from build123d import *

# Parameters (mm, degrees)
BOSS_EXTRUDE1_DEPTH = 17.5
FILLET1_R           = 2
SKETCH3_W           = 5
SKETCH3_H           = 7.5
CUT_EXTRUDE1_DEPTH  = 66


with BuildPart() as part:
    # Sketch2 → Boss-Extrude1 (new body, symmetric)
    with BuildSketch(Plane(origin=(0, 0, 0), x_dir=(1, 0, 0), z_dir=(0, 1, 0))):
        with BuildLine():
            Line((5.25, 14.75), (5.25, -14.75))
            ThreePointArc((5.25, -14.75), (0, -20), (5.25, -25.25))
            Line((5.25, -25.25), (5.25, -32.5))
            Line((5.25, -32.5), (-14.75, -32.5))
            Line((-14.75, -32.5), (-14.75, 32.5))
            Line((-14.75, 32.5), (5.25, 32.5))
            Line((5.25, 32.5), (5.25, 25.25))
            ThreePointArc((5.25, 25.25), (0, 20), (5.25, 14.75))
        make_face()
    extrude(amount=BOSS_EXTRUDE1_DEPTH, both=True)

    # Fillet1
    fillet1_edges = [part.edges().sort_by_distance(p)[0] for p in [
        (-14.75, -17.5, 0),
        (-4.75, -17.5, -32.5),
        (5.25, -17.5, -28.875),
        (0, -17.5, -20),
        (-4.75, 17.5, -32.5),
        (5.25, 0, 32.5),
        (-14.75, 0, 32.5),
        (-14.75, 0, -32.5),
        (5.25, 0, -32.5),
        (-14.75, 17.5, 0),
        (-4.75, 17.5, 32.5),
        (5.25, 17.5, 28.875),
        (0, 17.5, 20),
        (5.25, 17.5, 0),
        (0, 17.5, -20),
        (5.25, -17.5, 0),
        (5.25, 17.5, -28.875),
        (0, -17.5, 20),
        (5.25, -17.5, 28.875),
        (-4.75, -17.5, 32.5),
    ]]
    fillet(fillet1_edges, radius=FILLET1_R)

    # Sketch3 → Cut-Extrude1 (cut, through all)
    with BuildSketch(Plane.XY.offset(32.5)):
        with Locations((-12.25, 0)):
            Rectangle(SKETCH3_W, SKETCH3_H)
    extrude(amount=-CUT_EXTRUDE1_DEPTH, mode=Mode.SUBTRACT)


solid = part.part
Geometry: final body of the model. Coordinates: model frame, mm. A direction names the side the tool comes from. Give positions to 0.01 mm unless a question says otherwise; leave off trailing zeros. Write each loop counter-clockwise with the first axis right and the second up, starting at its lowest first coordinate (ties: lowest second). Pieces come first, ordered by that corner, then holes. Notation, with made-up numbers: (-30, 36) - (-2, 36) arc R20 ccw to (-2, 48) - close; hole circle Ø3 at (-10, 8.25). An arc over 180 degrees is marked (long way). Return JSON: item names as keys, results as strings. Group by question number.
1) Set-up query: faces 1 (the flat face through (-14.75, 10, 0)), 2 (the flat face through (-9.75, 0, 0)). Return all of +Z, -Z, +X, -X, +Y, -Y with unobstructed straight access to the full face (end or side cutting, diameter ignored); none if empty.
2) Section A-A on x = -11.5. Return the cut outline in (y, z).
3) Section D-D on y = -1. Return the cut outline in (x, z), plus the area to 3 significant figures.
4) First-contact query: P1, Ø4, axis at y = 1.5, z = -7.5, coming from the -X side. Flat tip, straight axial feed; report the tip coordinate or a pass-through.
5) Line query: line 1 (Z direction, x = 0.75, y = -12); line 2 (Z direction, x = 2.75, y = 8); line 3 (Y direction, x = -11.5, z = 18). Output: solid intervals per line, ascending.
6) Section B-B on z = -2. Return the cut outline in (x, y).
7) Section C-C on y = -6. Return the cut outline in (x, z).
Filled in:
{
 "1": {"face 1": "+Z, -Z, -X, +Y, -Y", "face 2": "+Z, -Z, -X"},
 "2": {"outline": "(-17.5, -30.5) arc R2 ccw to (-15.5, -32.5) - (-3.75, -32.5) - (-3.75, 32.5) - (-15.5, 32.5) arc R2 ccw to (-17.5, 30.5) - close; (3.75, -32.5) - (15.5, -32.5) arc R2 ccw to (17.5, -30.5) - (17.5, 30.5) arc R2 ccw to (15.5, 32.5) - (3.75, 32.5) - close"},
 "3": {"outline": "(-9.75, -32.5) - (3.25, -32.5) arc R2 ccw to (5.25, -30.5) - (5.25, -25.25) arc R5.25 cw to (5.25, -14.75) - (5.25, 14.75) arc R5.25 cw to (5.25, 25.25) - (5.25, 30.5) arc R2 ccw to (3.25, 32.5) - (-9.75, 32.5) - close", "area": "887 mm^2"},
 "4": {"P1": "stops at x = -9.75"},
 "5": {"line 1": "z = -32.5 to -22.7, -17.3 to 17.3, 22.7 to 32.5", "line 2": "z = -32.5 to -24.62, -15.38 to 15.38, 24.62 to 32.5", "line 3": "y = -17.5 to -3.75, 3.75 to 17.5"},
 "6": {"outline": "(-14.75, -15.5) arc R2 ccw to (-12.75, -17.5) - (3.25, -17.5) arc R2 ccw to (5.25, -15.5) - (5.25, 15.5) arc R2 ccw to (3.25, 17.5) - (-12.75, 17.5) arc R2 ccw to (-14.75, 15.5) - (-14.75, 3.75) - (-9.75, 3.75) - (-9.75, -3.75) - (-14.75, -3.75) - close"},
 "7": {"outline": "(-14.75, -30.5) arc R2 ccw to (-12.75, -32.5) - (3.25, -32.5) arc R2 ccw to (5.25, -30.5) - (5.25, -25.25) arc R5.25 cw to (5.25, -14.75) - (5.25, 14.75) arc R5.25 cw to (5.25, 25.25) - (5.25, 30.5) arc R2 ccw to (3.25, 32.5) - (-12.75, 32.5) arc R2 ccw to (-14.75, 30.5) - close"}
}
